from build123d import *

# Parameters (mm, degrees)
F0_R     = 139.7
F1_DEPTH = 50.8
F3_DEPTH = 50.801


with BuildPart() as f1:
    # F0 (on Top) → F1 (new body)
    with BuildSketch(Plane.XY):
        Circle(F0_R)
    extrude(amount=F1_DEPTH)

    # F2 (on face) → F3 (intersect, through all)
    with BuildSketch(Plane.XY.offset(50.8)):
        with BuildLine():
            Line((-81.829765289, 81.829765289), (-52.537943385, 103.1115196251))
            Line((-52.537943385, 103.1115196251), (-66.7753086177, 122.7075717265))
            ThreePointArc((-66.7753086177, 122.7075717265), (-82.1135997453, 113.0196741142), (-96.0671305217, 101.4258173904))
            Line((-96.0671305217, 101.4258173905), (-81.829765289, 81.829765289))
        make_face()
        with BuildLine():
            Line((-18.1033415291, 114.3), (18.1033415291, 114.3))
            Line((18.1033415291, 114.3), (18.1033415291, 138.522052488))
            ThreePointArc((18.1033415291, 138.522052488), (0, 139.7), (-18.1033415291, 138.522052488))
            Line((-18.1033415291, 138.522052488), (-18.1033415291, 114.3))
        make_face()
        with BuildLine():
            Line((52.537943385, 103.1115196251), (81.829765289, 81.829765289))
            Line((81.829765289, 81.829765289), (96.0671305217, 101.4258173905))
            ThreePointArc((96.0671305217, 101.4258173904), (82.1135997453, 113.0196741142), (66.7753086177, 122.7075717265))
            Line((66.7753086177, 122.7075717265), (52.537943385, 103.1115196251))
        make_face()
        with BuildLine():
            Line((103.1115196251, 52.537943385), (114.3, 18.1033415291))
            Line((114.3, 18.1033415291), (137.3365408567, 25.5883673865))
            ThreePointArc((137.3365408567, 25.5883673865), (132.8625953264, 43.1696741142), (126.1480604818, 60.0229692424))
            Line((126.1480604818, 60.0229692424), (103.1115196251, 52.537943385))
        make_face()
        with BuildLine():
            Line((137.3365408567, -25.5883673865), (114.3, -18.1033415291))
            Line((114.3, -18.1033415291), (103.1115196251, -52.537943385))
            Line((103.1115196251, -52.537943385), (126.1480604818, -60.0229692424))
            ThreePointArc((126.1480604818, -60.0229692424), (132.8625953264, -43.1696741142), (137.3365408567, -25.5883673865))
        make_face()
        with BuildLine():
            Line((96.0671305217, -101.4258173905), (81.829765289, -81.829765289))
            Line((81.829765289, -81.829765289), (52.537943385, -103.1115196251))
            Line((52.537943385, -103.1115196251), (66.7753086177, -122.7075717265))
            ThreePointArc((66.7753086177, -122.7075717265), (82.1135997453, -113.0196741142), (96.0671305217, -101.4258173904))
        make_face()
        with BuildLine():
            Line((18.1033415291, -138.522052488), (18.1033415291, -114.3))
            Line((18.1033415291, -114.3), (-18.1033415291, -114.3))
            Line((-18.1033415291, -114.3), (-18.1033415291, -138.522052488))
            ThreePointArc((-18.1033415291, -138.522052488), (0, -139.7), (18.1033415291, -138.522052488))
        make_face()
        with BuildLine():
            Line((-66.7753086177, -122.7075717265), (-52.537943385, -103.1115196251))
            Line((-52.537943385, -103.1115196251), (-81.829765289, -81.829765289))
            Line((-81.829765289, -81.829765289), (-96.0671305217, -101.4258173905))
            ThreePointArc((-96.0671305217, -101.4258173904), (-82.1135997453, -113.0196741142), (-66.7753086177, -122.7075717265))
        make_face()
        with BuildLine():
            Line((-126.1480604818, -60.0229692424), (-103.1115196251, -52.537943385))
            Line((-103.1115196251, -52.537943385), (-114.3, -18.1033415291))
            Line((-114.3, -18.1033415291), (-137.3365408567, -25.5883673865))
            ThreePointArc((-137.3365408567, -25.5883673865), (-132.8625953264, -43.1696741142), (-126.1480604818, -60.0229692424))
        make_face()
        with BuildLine():
            Line((-114.3, 18.1033415291), (-103.1115196251, 52.537943385))
            Line((-103.1115196251, 52.537943385), (-126.1480604818, 60.0229692424))
            ThreePointArc((-126.1480604818, 60.0229692424), (-132.8625953264, 43.1696741142), (-137.3365408567, 25.5883673865))
            Line((-137.3365408567, 25.5883673865), (-114.3, 18.1033415291))
        make_face()
        Polygon((114.3, -18.1033415291), (114.3, 18.1033415291), (103.1115196251, 52.537943385), (81.829765289, 81.829765289), (52.537943385, 103.1115196251), (18.1033415291, 114.3), (-18.1033415291, 114.3), (-52.537943385, 103.1115196251), (-81.829765289, 81.829765289), (-103.1115196251, 52.537943385), (-114.3, 18.1033415291), (-114.3, -18.1033415291), (-103.1115196251, -52.537943385), (-81.829765289, -81.829765289), (-52.537943385, -103.1115196251), (-18.1033415291, -114.3), (18.1033415291, -114.3), (52.537943385, -103.1115196251), (81.829765289, -81.829765289), (103.1115196251, -52.537943385), align=None)
    extrude(amount=-F3_DEPTH, mode=Mode.INTERSECT)


solid = f1.part
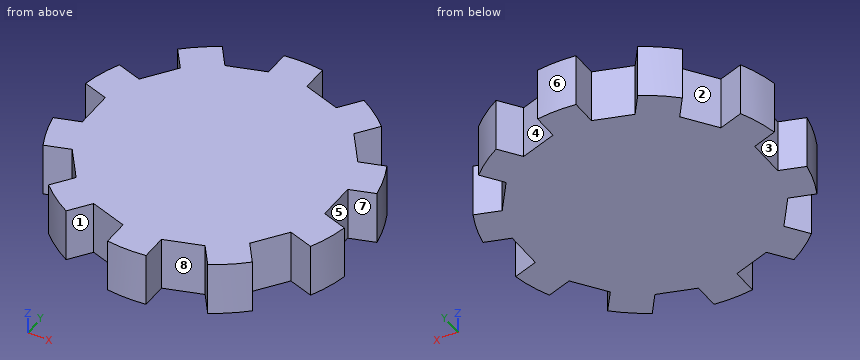
Source: CAD feature listing. Evaluate the final solid. Frame: model axes, mm. Face numbers are marked on the shaded views. A direction names the side the tool comes from. Coordinates: 2 decimals unless noted, no trailing zeros. Loops run counter-clockwise (first coordinate to the right, second up) from the corner with the lowest first, then second, coordinate; pieces in that order, holes last. Notation, with made-up numbers: (83.25, -35) -> (122.25, -35) arc R28 cw to (122.25, -8) -> close; hole circle Ø6 at (32.5, 57.25). An arc over 180 degrees is marked (long way). Answer in a Markdown table with one row per item. Add a question column.
Q1. Contact query for flat-ended pins moving along their axis: pin 1 Ø8 at (x, z) = (11.5, 20.5) entering from +Y; pin 2 Ø1 at (x, z) = (-43.5, 9) entering from +Y; pin 3 Ø19.5 at (y, z) = (-130.5, 22.5) entering from +X. Output: stop coordinate, or through.
Q2. Pull-direction query (X, two-part tool) for the marked faces 6, 7 and 8; classes: pulls with the +X half, pulls with the -X half, needs draft (parallel to the pull), parting line crosses it, or undercut.
Q3. Section C-C on x = 48. Return the cut outline in (y, z), and give its area (3 significant figures).
Q4. Section A-A on y = -107. Return the cut outline in (x, z).
Q5. Section B-B on x = 89.5. Return the cut outline in (y, z).
Q6. Ray query, line 1 along X through (y, z) = (116, 24.5); line 2 along Y through (x, z) = (-84, 26.5); line 3 along X through (y, z) = (127, 24). Return the intervals inside material, ascending.
Q7. Reachability of the marked faces 1, 2, 3, 4 and 5 from +Z, -Z, +X, -X, +Y, -Y: full face, straight path, thin tool, end or side. Return the list, or none.
Q8. Section D-D on y = -77.5. Return the cut outline in (x, z), and give its area (3 significant figures).
Computed values:
| question | item | result |
|---|---|---|
| 1 | pin 1 | stops at y = 139.5 |
| 1 | pin 2 | stops at y = 106.21 |
| 1 | pin 3 | stops at x = 70.25 |
| 2 | face 6 | parting line crosses it |
| 2 | face 7 | pulls with the +X half |
| 2 | face 8 | undercut |
| 3 | outline | (-104.59, 0) -> (104.59, 0) -> (104.59, 50.8) -> (-104.59, 50.8) -> close |
| 3 | area | 10,600 mm^2 |
| 4 | outline | (-89.82, 0) -> (-55.36, 0) -> (-55.36, 50.8) -> (-89.82, 50.8) -> close; (-40.57, 0) -> (40.57, 0) -> (40.57, 50.8) -> (-40.57, 50.8) -> close; (55.36, 0) -> (89.82, 0) -> (89.82, 50.8) -> (55.36, 50.8) -> close |
| 5 | outline | (-107.27, 0) -> (-92.39, 0) -> (-92.39, 50.8) -> (-107.27, 50.8) -> close; (-71.27, 0) -> (71.27, 0) -> (71.27, 50.8) -> (-71.27, 50.8) -> close; (92.39, 0) -> (107.27, 0) -> (107.27, 50.8) -> (92.39, 50.8) -> close |
| 6 | line 1 | x = -77.85 to -61.9, -18.1 to 18.1, 61.9 to 77.85 |
| 6 | line 2 | y = -111.62 to -84.82, -78.84 to 78.84, 84.82 to 111.62 |
| 6 | line 3 | x = -18.1 to 18.1 |
| 7 | face 1 | +Z, -Z, -Y |
| 7 | face 2 | +Z, -Z |
| 7 | face 3 | +Z, -Z, -X |
| 7 | face 4 | +Z, -Z, +Y |
| 7 | face 5 | +Z, -Z, +X |
| 8 | outline | (-84.98, 0) -> (84.98, 0) -> (84.98, 50.8) -> (-84.98, 50.8) -> close |
| 8 | area | 8,630 mm^2 |
